Geometry check sheet. Reference: drawing and pictorial views, mm from the part's lowest x, y, z. Coordinates: 2 decimals unless noted, no trailing zeros. Write each loop counter-clockwise with the first axis right and the second up, starting at its lowest first coordinate (ties: lowest second). Pieces come first, ordered by that corner, then holes. Notation, with made-up numbers: (-34.5, -21) - (-25.5, -21) arc R24 cw to (-25.5, 13) - close; hole circle Ø5 at (-1.75, 19). An arc over 180 degrees is marked (long way). Use one line per item in the form item = value. Start each with the question number.
(1) Gauge pin test, flat ends, axial feed: pin 1 Ø1.5 at (y, z) = (3.5, 16) entering from -X; pin 2 Ø1.5 at (x, z) = (4, 24) entering from -Y; pin 3 Ø2 at (y, z) = (1.5, 42) entering from -X (1 decimal). Record the tip position at first contact, or that the pin passes through.
(2) Sectioned sample at A-A (z = 67). Record the cut outline in (x, y) (1 decimal).
(3) Mould release check, pull along Z, two halves, no side actions. Record for the marked faces 1, 2 and 3: released by +Z, released by -Z, zero draft, split by the parting line, or undercut.
(4) Sectioned sample at B-B (z = 31). Record the cut outline in (x, y) (1 decimal).
(5) Material ranges on line 1 (Z direction, x = 6, y = 1.5); line 2 (Z direction, x = 4.75, y = 4.5); line 3 (X direction, y = 3, z = 14.5), recorded low to high. Write a range as [from, to].
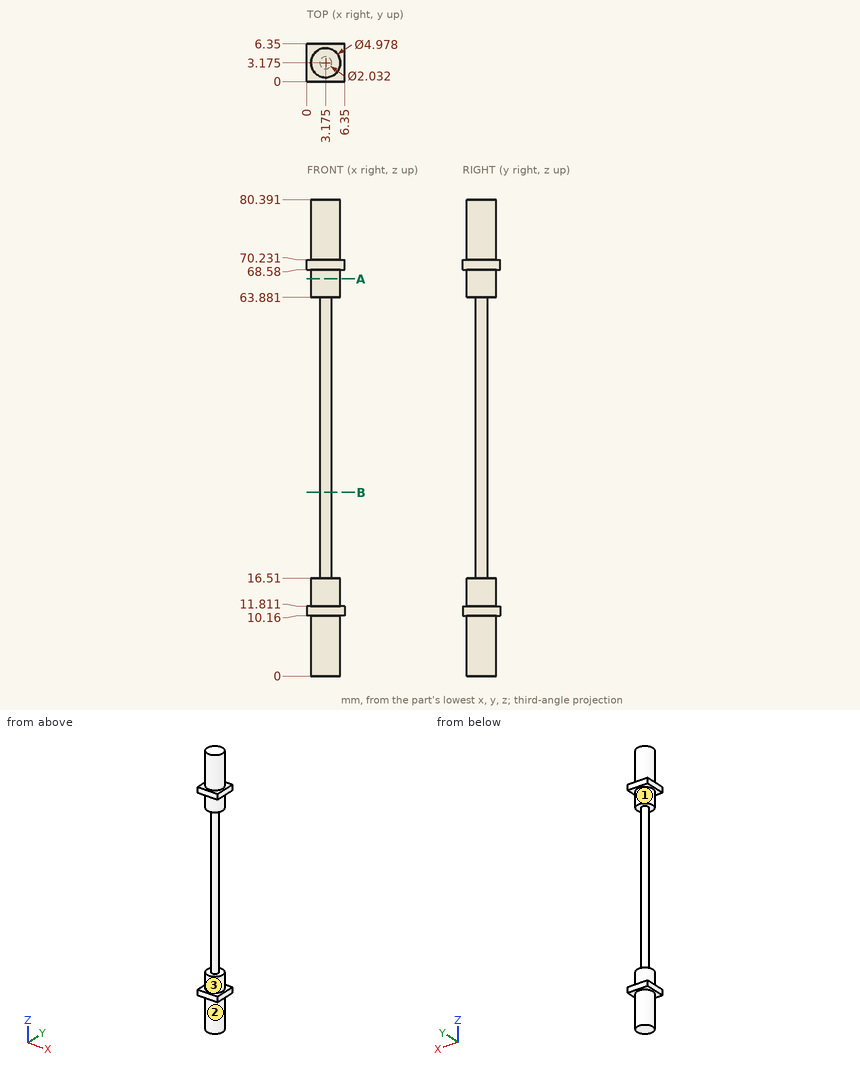
Answers below:
q1.pin_1 = 0.69
q1.pin_2 = 2.16
q1.pin_3 = 2.4
q2.outline = circle Ø5 at (3.2, 3.2)
q3.face_1 = undercut
q3.face_2 = zero draft
q3.face_3 = undercut
q4.outline = circle Ø2 at (3.2, 3.2)
q5.line_1 = [10.16, 11.81], [68.58, 70.23]
q5.line_2 = [0, 16.51], [63.88, 80.39]
q5.line_3 = [0.69, 5.66]
